Geometry: see drawing. Coordinates: mm, zero at the bounding-box minimum. A direction names the side the tool comes from. Give positions to 0.01 mm unless a question says otherwise; leave off trailing zeros. Write each loop counter-clockwise with the first axis right and the second up, starting at its lowest first coordinate (ties: lowest second). Pieces come first, ordered by that corner, then holes.
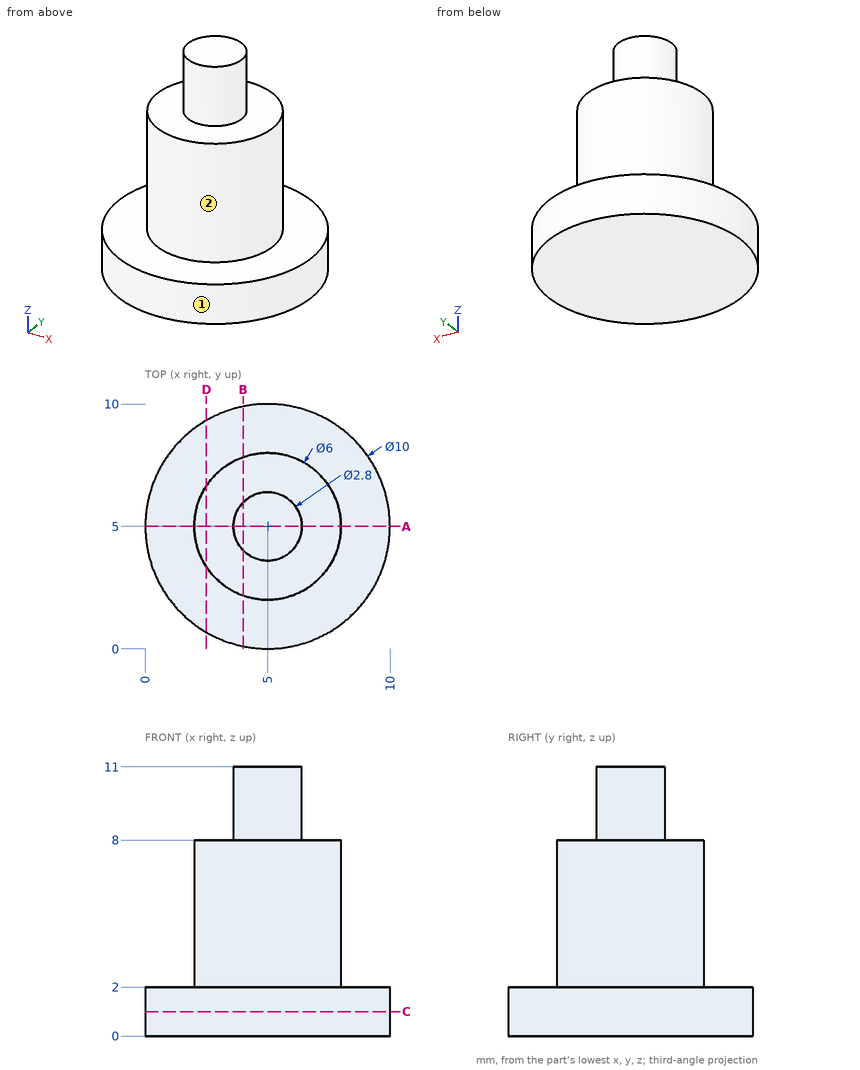
Q1. Pin query (flat end, axial travel): pin 1 (3 mm diameter, centred on y = 4.5, z = 4.5, fed in from -X); pin 2 (1 mm diameter, centred on x = 7.5, z = 4.5, fed in from +Y); pin 3 (4 mm diameter, centred on y = 7, z = 9.5, fed in from -X). Return the tip coordinate at first contact, or that it passes through.
Q2. Access query for the marked faces 1 and 2. Directions: +Z, -Z, +X, -X, +Y, -Y. A direction counts if a zero-diameter tool reaches every point of the face in a straight line with its end or side. Return the directions, or none.
Q3. Material intervals for line 1 along Z through (x, y) = (3.75, 6); line 2 along Z through (x, y) = (3.25, 2.5); line 3 along X through (y, z) = (3, 3.75), sorted ascending.
Q4. Section D-D, the plane x = 2.5. Return the cut outline in (y, z), then the cut area to 3 significant figures.
Q5. Section B-B, the plane x = 4. Return the cut outline in (y, z).
Q6. Section C-C, the plane z = 1. Return the cut outline in (x, y), then the cut area to 3 significant figures.
Q7. Section A-A, the plane y = 5. Return the cut outline in (x, z), then the cut area to 3 significant figures.
Solutions:
1. pin 1: stops at x = 2
1. pin 2: stops at y = 7.24
1. pin 3: stops at x = 2.08
2. face 1: +Z, -Z
2. face 2: +Z
3. line 1: z = 0 to 8
3. line 2: z = 0 to 2
3. line 3: x = 2.76 to 7.24
4. outline: (0.67, 0) - (9.33, 0) - (9.33, 2) - (6.66, 2) - (6.66, 8) - (3.34, 8) - (3.34, 2) - (0.67, 2) - close
4. area: 37.2 mm2
5. outline: (0.1, 0) - (9.9, 0) - (9.9, 2) - (7.83, 2) - (7.83, 8) - (5.98, 8) - (5.98, 11) - (4.02, 11) - (4.02, 8) - (2.17, 8) - (2.17, 2) - (0.1, 2) - close
6. outline: circle Ø10 at (5, 5)
6. area: 78.5 mm2
7. outline: (0, 0) - (10, 0) - (10, 2) - (8, 2) - (8, 8) - (6.4, 8) - (6.4, 11) - (3.6, 11) - (3.6, 8) - (2, 8) - (2, 2) - (0, 2) - close
7. area: 64.4 mm2
